Model file for the job. Use its own axes, mm. A direction names the side the tool comes from. Coordinates: 2 decimals unless noted, no trailing zeros. Loops run counter-clockwise (first coordinate to the right, second up) from the corner with the lowest first, then second, coordinate; pieces in that order, holes last. Notation, with made-up numbers: (48.25, -37) - (93.25, -37) arc R19 ccw to (93.25, -18) - close; hole circle Ø7 at (7.5, -39). An arc over 180 degrees is marked (long way). Write each question's results on one line, items separated by ' | '. Start each with the question number.
Autodesk Inventor part; units mm, degrees
ref_plane "YZ Plane" through (0, 0, 0) normal (1, 0, 0) x (0, 1, 0)
ref_plane "XZ Plane" through (0, 0, 0) normal (0, 1, 0) x (-1, 0, 0)
ref_plane "XY Plane" through (0, 0, 0) normal (0, 0, 1) x (1, 0, 0)
sketch "Sketch1" plane through (0, 0, 0) normal (0, 0, 1) x (1, 0, 0)
  circle A0 centre (-0.9126, 2.0208) radius 3.175
  circle A1 centre (-0.9126, 2.0208) radius 6.35
  point P0 (0, 0)
  dimension "d0" = 6.35
  dimension "d1" = 12.7
extrude "Extrusion1" add sketch "Sketch1" along normal blind 25.4
sketch "Sketch2" plane through (-0.9126, 2.0208, 25.4) normal (0, 0, 1) x (1, 0, 0)
  line L0 (-3.2261, 4.7402) -> (3.0392, 4.7402)
  line L1 (3.0392, 4.7402) -> (3.0392, 2.5812)
  line L2 (3.0392, 2.5812) -> (-3.2261, 2.5812)
  line L3 (-3.2261, 2.5812) -> (-3.2261, 4.7402)
  point P0 (0.9126, -2.0208)
  dimension "d6" = 2.159
extrude "Extrusion2" add sketch "Sketch2" against normal blind 25.4
sketch "Sketch3" plane through (-0.9126, 2.0208, 25.4) normal (0, 0, 1) x (1, 0, 0)
  circle A0 centre (0, 0) radius 6.35
  point P0 (0.9126, -2.0208)
extrude "Extrusion3" add sketch "Sketch3" along normal blind 101.6
properties part number "motoradaptor"
Q1. Cut at C-C (z = 119.5). List the corners of the cut face in (x, y).
Q2. Mould opens along Y. For faces 3 (the cylindrical face through (-0.801, -1.152, 12.522)), 4 (the flat face through (-1, 4.602, 13)), 5 (the cylindrical face through (-1.739, -4.275, 62.611)), 6 (the flat face through (-1, 5, 0)) say: +Y half, -Y half, draft (parallel to the pull), parting line (faces both ways), or undercut.
Q3. Cut at A-A (x = -0.75). List the corners of the cut face in (y, z).
Q4. Drill centre lines: L1, parallel to Z at x = -1.75, y = 0; L2, parallel to Y at x = -1.25, z = 29; L3, parallel to X at y = 4.75, z = 64.5. Where is each one in solid material? Low to high. Write a range as from..to.
Q5. Which spindle directions (+Z, -Z, +X, -X, +Y, -Y) get a long thin tool onto all of the face, cutting with end or side? Do faces 1 (the flat face through (-1, 2, 127)), 2 (the flat face through (-1, 2, 25.4)). Say none if no direction does.
Q6. Cut at D-D (y = 6.5). List the corners of the cut face in (x, z), and give its area (3 significant figures).
Q7. Cut at B-B (y = 0.5). List the corners of the cut face in (x, z), and give its area (3 significant figures).
Q8. Pin check, flat tips, straight feed: pin 1 (1.5 mm diameter, centred on x = -2.5, z = 52, fed in from -Y); pin 2 (1 mm diameter, centred on y = 0, z = 91.5, fed in from -X); pin 3 (5 mm diameter, centred on y = -1.5, z = 16, fed in from -X). Stop position of each tip, or through.
Check result:
1) outline: circle Ø12.7 at (-0.91, 2.02)
2) face 3: undercut | face 4: undercut | face 5: parting line | face 6: draft
3) outline: (-4.33, 0) - (-1.15, 0) - (-1.15, 25.4) - (4.6, 25.4) - (4.6, 0) - (8.37, 0) - (8.37, 127) - (-4.33, 127) - close
4) L1: 25.4..127 | L2: -4.32..8.36 | L3: -6.65..4.82
5) face 1: +Z, +X, -X, +Y, -Y | face 2: -Z
6) outline: (-5.41, 0) - (3.59, 0) - (3.59, 127) - (-5.41, 127) - close | area: 1,140 mm²
7) outline: (-7.08, 0) - (-3.7, 0) - (-3.7, 25.4) - (1.87, 25.4) - (1.87, 0) - (5.25, 0) - (5.25, 127) - (-7.08, 127) - close | area: 1,420 mm²
8) pin 1: y = -4.27 | pin 2: x = -7.08 | pin 3: x = -7.18
